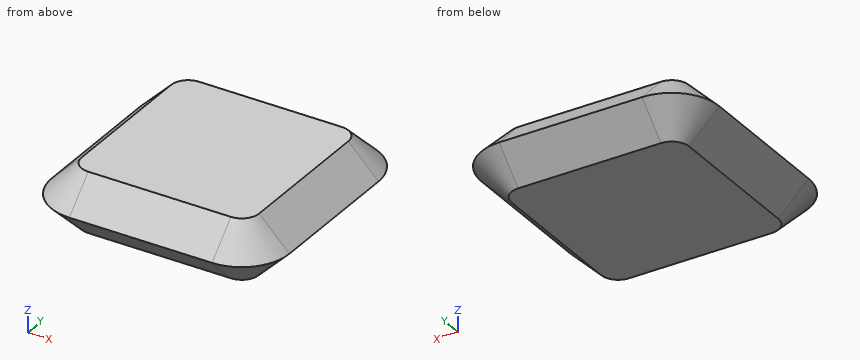
```python
from build123d import *

# Parameters (mm, degrees)
F1_DEPTH = 25.4
F2_SIZE  = 12.7
F3_SIZE  = 12.69999


# Not quite as in the source:
# - a fillet or chamfer is up to 0.001 mm smaller than in the source, because OpenCascade refuses the exact size


with BuildPart() as f1:
    # F0 (on Top) → F1 (new body)
    with BuildSketch(Plane.XY):
        with BuildLine():
            Line((-30, -50), (30, -50))
            ThreePointArc((30, -50), (44.1421356237, -44.1421356237), (50, -30))
            Line((50, -30), (50, 30))
            ThreePointArc((50, 30), (44.1421356237, 44.1421356237), (30, 50))
            Line((30, 50), (-30, 50))
            ThreePointArc((-30, 50), (-44.1421356237, 44.1421356237), (-50, 30))
            Line((-50, 30), (-50, -30))
            ThreePointArc((-50, -30), (-44.1421356237, -44.1421356237), (-30, -50))
        make_face()
    extrude(amount=F1_DEPTH)

    # F2
    f2_edges = [f1.edges().sort_by_distance(p)[0] for p in [
        (0, -50, 25.4),
        (44.142136, -44.142136, 25.4),
        (50, 0, 25.4),
        (44.142136, 44.142136, 25.4),
        (0, 50, 25.4),
        (-44.142136, 44.142136, 25.4),
        (-50, 0, 25.4),
        (-44.142136, -44.142136, 25.4),
    ]]
    chamfer(f2_edges, length=F2_SIZE)

    # F3 (size 12.7 in the source; OpenCascade refuses exactly that, so slightly less here)
    f3_edges = [f1.edges().sort_by_distance(p)[0] for p in [
        (0, -50, 0),
        (44.142136, -44.142136, 0),
        (50, 0, 0),
        (44.142136, 44.142136, 0),
        (0, 50, 0),
        (-44.142136, 44.142136, 0),
        (-50, 0, 0),
        (-44.142136, -44.142136, 0),
    ]]
    chamfer(f3_edges, length=F3_SIZE)


solid = f1.part
```
Input: part model. Units: mm. Frame: model coordinates. Give positions to 0.01 mm unless a question says otherwise; leave off trailing zeros. Order: outer loops, then holes, each group sorted by start corner. A loop starts at its lowest first (then second) coordinate and runs counter-clockwise, first axis right, second up. Notation, with made-up numbers: M -33,30 L 17,30 A29 ccw 17,61 Z; hole C 84,32 d1. An arc over 180 degrees is marked long. One line per question, with ' | ' between items. Start each with the question number.
1. Material intervals for probe 1 along Y at (x, z) = (33.5, 4); probe 2 along X at (y, z) = (-31, 6.25); probe 3 along X at (y, z) = (29, 19.75), sorted ascending. Write a range as [from, to].
2. First-contact query: pin 1 Ø4 at (x, z) = (34, 15) entering from +Y; pin 2 Ø1.5 at (y, z) = (26, 21.5) entering from +X; pin 3 Ø1.5 at (x, z) = (-13, 15.5) entering from +Y; pin 4 Ø10 at (x, y) = (-8, -33.5) entering from -Z. Flat tips, straight axial feed; report the tip coordinate or a pass-through.
3. Section query B-B (z = 15.5). Return the cut outline in (x, y).
Here are the results:
1) probe 1: [-40.74, 40.74] | probe 2: [-43.51, 43.51] | probe 3: [-42.95, 42.95]
2) pin 1: y = 49.33 | pin 2: x = 41.95 | pin 3: y = 47.95 | pin 4: z = 0
3) outline: M -47.2,-30 A17.2 ccw -30,-47.2 L 30,-47.2 A17.2 ccw 47.2,-30 L 47.2,30 A17.2 ccw 30,47.2 L -30,47.2 A17.2 ccw -47.2,30 Z
